Autodesk Inventor part; units mm, degrees
ref_plane "YZ Plane" through (0, 0, 0) normal (1, 0, 0) x (0, 1, 0)
ref_plane "XZ Plane" through (0, 0, 0) normal (0, 1, 0) x (-1, 0, 0)
ref_plane "XY Plane" through (0, 0, 0) normal (0, 0, 1) x (1, 0, 0)
sketch "Sketch1" plane through (0, 0, 0) normal (0, 0, 1) x (1, 0, 0)
  line L0 (0, -2.2666) -> (0, 12.7444)
  line L1 (0, 10.6) -> (0, 0.59)
  line L2 (8.9, 0) -> (8.9, 0.82)
  line L3 (8.9, 0.82) -> (1.41, 0.82)
  line L4 (0.82, 1.41) -> (0.82, 10.6)
  line L5 (0, 10.6) -> (0.82, 10.6)
  line L6 (0.59, 0) -> (8.9, 0)
  arc A0 (0.82, 1.41) -> (1.41, 0.82) centre (1.41, 1.41) ccw
  arc A1 (0, 0.59) -> (0.59, 0) centre (0.59, 0.59) ccw
  point P0 (0, 0)
  dimension "d0" = 10.6
  dimension "d1" = 8.9
  dimension "d2" = 0.82
  dimension "d3" = 0.82
  dimension "d4" = 0.59
extrude "Extrusion1" add sketch "Sketch1" along normal blind 7.2
sketch "Sketch2" plane through (1.41, 0.82, 0) normal (0, 1, 0) x (1, 0, 0)
  line L0 (0, -7.2) -> (7.49, -7.2)
  circle A0 centre (3.99, -3.6) radius 1.6
  line L1 (7.49, 0) -> (7.49, -7.2)
  point P0 (-1.41, 0)
  dimension "d7" = 3.5
  dimension "d8" = 3.2
  dimension "d9" = 3.6
extrude "Extrusion2" cut sketch "Sketch2" against normal through all
sketch "Sketch3" plane through (0.82, 1.41, 0) normal (1, 0, 0) x (0, 0, -1)
  line L0 (0, 0) -> (0, 9.19)
  line L1 (0, 9.19) -> (-7.2, 9.19)
  circle A0 centre (-3.6, 5.69) radius 1.825
  point P0 (0, -1.41)
  dimension "d12" = 3.65
  dimension "d13" = 3.5
  dimension "d14" = 3.6
extrude "Extrusion3" cut sketch "Sketch3" against normal through all
properties part number "LCouplerSmall"
Build history of the part. All positions in model axes, mm. A direction names the side the tool comes from. Round coordinates to 2 decimals unless told otherwise and drop trailing zeros. Write each loop counter-clockwise with the first axis right and the second up, starting at its lowest first coordinate (ties: lowest second). Pieces come first, ordered by that corner, then holes. Notation, with made-up numbers: M -16.75,50 L 18.25,50 A31 ccw 18.25,89 Z; hole C 20.25,-20 d5. An arc over 180 degrees is marked long. Use CSV: the item, a comma, the result in double quotes.
1. Saw through at C-C (x = 5.4). Give the cut face in (y, z).
Reply:
outline,"M 0,0 L 0.82,0 L 0.82,2 L 0,2 Z; M 0,5.2 L 0.82,5.2 L 0.82,7.2 L 0,7.2 Z"
2. Tool access for faces 1 (the face through (0.4, 10.6, 3.5)), 2 (the face through (0.82, 5, 4)): list every direction of +Z, -Z, +X, -X, +Y, -Y with a clear straight run to the whole face (end or side of a thin tool).
Reply:
face 1,"+Z, -Z, +X, -X, +Y"
face 2,"+Z, -Z, +X, +Y"
3. Two-plate mould, pull along X, no slides. Class faces 3 (the face through (0, 4, 4)), 4 (the face through (5.05, 0.42, 5.16)), 5 (the face through (8.9, 0.4, 3.5)), 6 (the face through (0.5, 3.4, 0)): +X half, -X half, draft (parallel to the pull), parting line (faces both ways), or undercut.
Reply:
face 3,"-X half"
face 4,"undercut"
face 5,"+X half"
face 6,"draft"
4. Saw through at D-D (x = 2.5). Give the cut face in (y, z).
Reply:
outline,"M 0,0 L 0.82,0 L 0.82,7.2 L 0,7.2 Z"
5. Flat gauge pins, fed straight in: pin 1 (3.5 mm diameter, centred on x = 5.5, z = 3, fed in from +Y); pin 2 (1 mm diameter, centred on x = 7, z = 5.5, fed in from -Y). Where does each tip first touch, or does it go through?
Reply:
pin 1,"stops at y = 0.82"
pin 2,"stops at y = 0"
6. Wall check: probe 1 along Z at (x, y) = (5.4, 0.65); probe 2 along Y at (x, z) = (4, 2). Give the ranges that are in metal, low to high. Write a range as from..to.
Reply:
probe 1,"z = 0..2, 5.2..7.2"
probe 2,"y = 0..0.82"
7. Saw through at B-B (y = 7.1). Give the cut face in (x, z) (3 decimals), plus the area to 3 significant figures.
Reply:
outline,"M 0,0 L 0.82,0 L 0.82,1.775 L 0,1.775 Z; M 0,5.425 L 0.82,5.425 L 0.82,7.2 L 0,7.2 Z"
area,"2.91 mm²"
8. Saw through at A-A (z = 3.6). Give the cut face in (x, y) (3 decimals).
Reply:
outline,"M 0,0.59 A0.59 ccw 0.59,0 L 3.8,0 L 3.8,0.82 L 1.41,0.82 A0.59 cw 0.82,1.41 L 0.82,5.275 L 0,5.275 Z; M 0,8.925 L 0.82,8.925 L 0.82,10.6 L 0,10.6 Z; M 7,0 L 8.9,0 L 8.9,0.82 L 7,0.82 Z"
